from build123d import *

# Parameters (mm, degrees)
F0_R     = 4
F0_R_2   = 75
F0_R_3   = 4.7625
F0_R_4   = 22.225
F1_DEPTH = 3.175


with BuildPart() as f1:
    # F0 (on Front) → F1 (new body)
    with BuildSketch(Plane.XZ):
        Polygon((-140.838728, 148.5138), (-140.838728, -72.2862), (347.514372, -72.2862), (347.514372, 38.1), (347.514372, 148.5138), align=None)
        with Locations((-115.438728, -46.8862)):
            Circle(F0_R, mode=Mode.SUBTRACT)
        with Locations((54.561272, -46.8862)):
            Circle(F0_R, mode=Mode.SUBTRACT)
        with Locations((-30.437628, 38.1)):
            Circle(F0_R_2, mode=Mode.SUBTRACT)
        with Locations((296.714372, 0)):
            Circle(F0_R_3, mode=Mode.SUBTRACT)
        with Locations((296.714372, 38.1)):
            Circle(F0_R_4, mode=Mode.SUBTRACT)
        with Locations((-115.438728, 123.1138)):
            Circle(F0_R, mode=Mode.SUBTRACT)
        with Locations((54.561272, 123.1138)):
            Circle(F0_R, mode=Mode.SUBTRACT)
        with Locations((296.714372, 76.2)):
            Circle(F0_R_3, mode=Mode.SUBTRACT)
    extrude(amount=F1_DEPTH)


solid = f1.part
CAD build for the part. Positions are in the model's coordinates, mm. Round coordinates to 2 decimals unless told otherwise and drop trailing zeros. Write each loop counter-clockwise with the first axis right and the second up, starting at its lowest first coordinate (ties: lowest second). Pieces come first, ordered by that corner, then holes. Notation, with made-up numbers: M -14,53.5 L -3,53.5 A26 cw -3,67.5 Z; hole C -16,9.25 d5. An arc over 180 degrees is marked long. Use a Markdown table: item, result. Add a question column.
1. Slice it at A-A on z = 38.1. Give the cut face in (x, y) (3 decimals), then the cut area to 3 significant figures.
2. Slice it at C-C on y = -1.6. Give the number of separate pieces and of enclosed holes in the cut face, then the cut area to 3 significant figures.
3. Slice it at B-B on x = 308.5. Give the cut face in (y, z) (3 decimals).
4. Slice it at D-D on z = 0. Give the cut face in (x, y) (3 decimals).
5. Pull direction X, two halves, no side cores. Call faces 1 (the face through (41.1, -1.57, 60.63)), 2 (the face through (100, 0, 40)): released by +X, released by -X, zero draft, split by the parting line, or undercut.
6. Flat gauge pin, fed straight in: P1, Ø8.5, axis at x = 296.71, z = 76.2, coming from the -Y side. Where does the tip first touch, or does it go through?
7. Drill centre lines: probe 1 along X at (y, z) = (-0.2, 123); probe 2 along X at (y, z) = (-2.1, 72.5); probe 3 along Z at (x, y) = (-68.5, -2.2). Where is each one in solid material? Low to high.
Reply:
| question | item | result |
|---|---|---|
| 1 | outline | M -140.839,-3.175 L -105.438,-3.175 L -105.438,0 L -140.839,0 Z; M 44.562,-3.175 L 274.489,-3.175 L 274.489,0 L 44.562,0 Z; M 318.939,-3.175 L 347.514,-3.175 L 347.514,0 L 318.939,0 Z |
| 1 | area | 933 mm^2 |
| 2 | separate pieces | 1 |
| 2 | enclosed holes | 8 |
| 2 | area | 88,300 mm^2 |
| 3 | outline | M -3.175,-72.286 L 0,-72.286 L 0,19.257 L -3.175,19.257 Z; M -3.175,56.943 L 0,56.943 L 0,148.514 L -3.175,148.514 Z |
| 4 | outline | M -140.839,-3.175 L -95.039,-3.175 L -95.039,0 L -140.839,0 Z; M 34.164,-3.175 L 291.952,-3.175 L 291.952,0 L 34.164,0 Z; M 301.477,-3.175 L 347.514,-3.175 L 347.514,0 L 301.477,0 Z |
| 5 | face 1 | undercut |
| 5 | face 2 | zero draft |
| 6 | P1 | passes through |
| 7 | probe 1 | x = -140.84 to -119.44, -111.44 to 50.56, 58.56 to 347.51 |
| 7 | probe 2 | x = -140.84 to -97.08, 36.21 to 293.72, 299.71 to 347.51 |
| 7 | probe 3 | z = -72.29 to -26.52, 102.72 to 148.51 |
